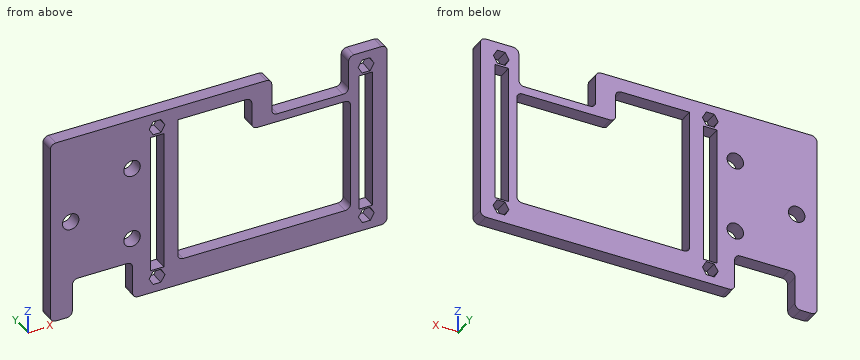
Autodesk Inventor part; units mm, degrees
ref_plane "YZ Plane" through (0, 0, 0) normal (1, 0, 0) x (0, 1, 0)
ref_plane "XZ Plane" through (0, 0, 0) normal (0, 1, 0) x (-1, 0, 0)
ref_plane "XY Plane" through (0, 0, 0) normal (0, 0, 1) x (1, 0, 0)
sketch "Sketch1" plane through (0, 0, 0) normal (0, 1, 0) x (-1, 0, 0)
  line L0 (-2.27, 0) -> (120.44, 0)
  line L1 (120.44, 0) -> (120.44, -68.57)
  line L2 (120.44, -68.57) -> (-2.27, -68.57)
  line L3 (-2.27, -68.57) -> (-2.27, 0)
  line L4 (120.44, -66.57) -> (120.44, -2)
  line L5 (0, -68.57) -> (118.44, -68.57)
  line L6 (-2.27, -2.27) -> (-2.27, -66.3)
  circle A0 centre (81.55, -63.09) radius 1.5
  circle A1 centre (81.55, -63.09) radius 1.5
  line L7 (70.44, -68.57) -> (15.73, -68.57)
  line L8 (51, 0) -> (75, 0)
  line L9 (26, 0) -> (51, 0)
  line L10 (84, -60) -> (79, -60)
  line L11 (79, -60) -> (79, -8.7337)
  line L12 (79, -8.7337) -> (84, -8.7337)
  line L13 (84, -8.7337) -> (84, -60)
  line L14 (8, -60) -> (3, -60)
  line L15 (3, -60) -> (3, -8.7337)
  line L16 (3, -8.7337) -> (8, -8.7337)
  line L17 (8, -8.7337) -> (8, -60)
  circle A2 centre (5.25, -63.09) radius 1.5
  circle A3 centre (5.35, -5.47) radius 1.5
  circle A4 centre (81.55, -5.47) radius 1.5
  circle A5 centre (81.55, -5.47) radius 1.5
  circle A6 centre (5.35, -5.47) radius 1.5
  circle A7 centre (5.25, -63.09) radius 1.5
  dimension "d20" = 3
  dimension "d27" = 3
  dimension "d28" = 3
  dimension "d29" = 3
  dimension "d30" = 68.57
extrude "Extrusion1" add sketch "Sketch1" along normal blind 5
fillet "Fillet4" radius 2 4 edges at (-120.44, 2.5, -68.57) (-120.44, 2.5, 0) (2.27, 2.5, -68.57) (2.27, 2.5, 0)
sketch "Sketch7" plane through (0, 5, 0) normal (0, 1, 0) x (1, 0, 0)
  line L0 (-117.44, 63.57) -> (-87.44, 63.57)
  line L1 (-87.44, 63.57) -> (-87.44, 5)
  line L2 (-87.44, 5) -> (-117.44, 5)
  line L3 (-117.44, 5) -> (-117.44, 63.57)
  line L4 (-120.44, 66.57) -> (-120.44, 2)
  line L5 (0.27, 68.57) -> (-118.44, 68.57)
  line L6 (-118.44, 0) -> (0.27, 0)
  point P0 (0, 0)
  dimension "d67" = 30
  dimension "d68" = 3
  dimension "d69" = 5
  dimension "d70" = 5
extrude "Extrusion6" [suppressed]
fillet "Fillet8" [suppressed]
sketch "Sketch8" plane through (0, 5, 0) normal (0, 1, 0) x (1, 0, 0)
  line L0 (-118.44, 0) -> (0.27, 0)
  line L1 (-39.73, 0) -> (-11.73, 0)
  line L2 (-11.73, 0) -> (-11.73, 14)
  line L3 (-11.73, 14) -> (-39.73, 14)
  line L4 (-39.73, 14) -> (-39.73, 0)
  line L5 (2.27, 2) -> (2.27, 66.57)
  point P0 (0, 0)
  point P1 (-11.73, 0)
  dimension "d74" = 28
  dimension "d75" = 14
  dimension "d82" = 14
extrude "Extrusion7" cut sketch "Sketch8" against normal blind 10
sketch "Sketch9" plane through (0, 5, 0) normal (0, 1, 0) x (1, 0, 0)
  line L0 (-74, 59) -> (-11, 59)
  line L1 (-11, 59) -> (-11, 17)
  line L2 (-11, 17) -> (-74, 17)
  line L3 (-74, 17) -> (-74, 59)
  line L4 (-74, 17) -> (-47.019, 17)
  line L5 (-47.019, 17) -> (-47.019, 5)
  line L6 (-47.019, 5) -> (-74, 5)
  line L7 (-74, 5) -> (-74, 17)
  point P0 (0, 0)
extrude "Extrusion8" cut sketch "Sketch9" against normal blind 5
fillet "Fillet9" radius 2 5 edges at (-74, 2.5, -59) (-11, 2.5, -59) (-11, 2.5, -17) (-47.019, 2.5, -5) (-47.019, 2.5, -17)
fillet "Fillet10" radius 2 4 edges at (-39.73, 2.5, -14) (-11.73, 2.5, -14) (-11.73, 2.5, 0) (-39.73, 2.5, 0)
sketch "Sketch10" plane through (0, 0, 0) normal (0, -1, 0) x (1, 0, 0)
  circle A0 centre (-90.66, -18.55) radius 3
  circle A1 centre (-113.03, -32.07) radius 3
  circle A2 centre (-90.66, -45.53) radius 3
  line L0 (-120.44, -66.57) -> (-120.44, -2)
  line L1 (-118.44, 0) -> (-41.73, 0)
  line L2 (-90.66, -45.53) -> (-90.66, -18.55) construction
  point P0 (0, 0)
  dimension "d83" = 29.78
  dimension "d84" = 18.55
  dimension "d85" = 6
  dimension "d86" = 13.52
  dimension "d87" = 6
  dimension "d88" = 22.37
  dimension "d89" = 13.46
  dimension "d90" = 6
extrude "Extrusion9" cut sketch "Sketch10" against normal blind 10
sketch "Sketch11" plane through (0, 0, 0) normal (0, -1, 0) x (1, 0, 0)
  circle A0 centre (-90.66, -18.55) radius 3
  line L0 (-92.9694, -18.55) -> (-91.8147, -16.55)
  line L1 (-91.8147, -16.55) -> (-89.5053, -16.55)
  line L2 (-89.5053, -16.55) -> (-88.3506, -18.55)
  line L3 (-88.3506, -18.55) -> (-89.5053, -20.55)
  line L4 (-89.5053, -20.55) -> (-91.8147, -20.55)
  line L5 (-91.8147, -20.55) -> (-92.9694, -18.55)
  circle A1 centre (-113.03, -32.07) radius 3
  line L6 (-115.3394, -32.07) -> (-114.1847, -30.07)
  line L7 (-114.1847, -30.07) -> (-111.8753, -30.07)
  line L8 (-111.8753, -30.07) -> (-110.7206, -32.07)
  line L9 (-110.7206, -32.07) -> (-111.8753, -34.07)
  line L10 (-111.8753, -34.07) -> (-114.1847, -34.07)
  line L11 (-114.1847, -34.07) -> (-115.3394, -32.07)
  circle A2 centre (-90.66, -45.53) radius 3
  line L12 (-92.9694, -45.53) -> (-91.8147, -43.53)
  line L13 (-91.8147, -43.53) -> (-89.5053, -43.53)
  line L14 (-89.5053, -43.53) -> (-88.3506, -45.53)
  line L15 (-88.3506, -45.53) -> (-89.5053, -47.53)
  line L16 (-89.5053, -47.53) -> (-91.8147, -47.53)
  line L17 (-91.8147, -47.53) -> (-92.9694, -45.53)
  point P0 (0, 0)
  dimension "d93" = 4
  dimension "d94" = 4
  dimension "d95" = 4
extrude "Extrusion10" [suppressed]
sketch "Sketch12" plane through (0, 0, 0) normal (0, -1, 0) x (1, 0, 0)
  circle A0 centre (-5.35, -5.47) radius 1.5
  line L0 (-8.2368, -5.47) -> (-6.7934, -2.97)
  line L1 (-6.7934, -2.97) -> (-3.9066, -2.97)
  line L2 (-3.9066, -2.97) -> (-2.4632, -5.47)
  line L3 (-2.4632, -5.47) -> (-3.9066, -7.97)
  line L4 (-3.9066, -7.97) -> (-6.7934, -7.97)
  line L5 (-6.7934, -7.97) -> (-8.2368, -5.47)
  circle A1 centre (-81.55, -5.47) radius 1.5
  line L6 (-84.4368, -5.47) -> (-82.9934, -2.97)
  line L7 (-82.9934, -2.97) -> (-80.1066, -2.97)
  line L8 (-80.1066, -2.97) -> (-78.6632, -5.47)
  line L9 (-78.6632, -5.47) -> (-80.1066, -7.97)
  line L10 (-80.1066, -7.97) -> (-82.9934, -7.97)
  line L11 (-82.9934, -7.97) -> (-84.4368, -5.47)
  circle A2 centre (-81.55, -63.09) radius 1.5
  line L12 (-84.4368, -63.09) -> (-82.9934, -60.59)
  line L13 (-82.9934, -60.59) -> (-80.1066, -60.59)
  line L14 (-80.1066, -60.59) -> (-78.6632, -63.09)
  line L15 (-78.6632, -63.09) -> (-80.1066, -65.59)
  line L16 (-80.1066, -65.59) -> (-82.9934, -65.59)
  line L17 (-82.9934, -65.59) -> (-84.4368, -63.09)
  circle A3 centre (-5.25, -63.09) radius 1.5
  line L18 (-6.6934, -60.59) -> (-3.8066, -60.59)
  line L19 (-3.8066, -60.59) -> (-2.3632, -63.09)
  line L20 (-2.3632, -63.09) -> (-3.8066, -65.59)
  line L21 (-3.8066, -65.59) -> (-6.6934, -65.59)
  line L22 (-6.6934, -65.59) -> (-8.1368, -63.09)
  line L23 (-8.1368, -63.09) -> (-6.6934, -60.59)
  line L24 (-8, -60) -> (-3, -60)
  line L25 (-84, -60) -> (-79, -60)
  line L26 (-79, -8.7337) -> (-84, -8.7337)
  line L27 (-3, -8.7337) -> (-8, -8.7337)
  point P0 (0, 0)
  dimension "d98" = 5
  dimension "d99" = 5
  dimension "d100" = 5
extrude "Extrusion11" cut sketch "Sketch12" against normal blind 10
sketch "Sketch13" plane through (0, 5, 0) normal (0, 1, 0) x (1, 0, 0)
  line L0 (0.27, 68.57) -> (-118.44, 68.57)
  line L1 (-112.44, 68.57) -> (-90.44, 68.57)
  line L2 (-90.44, 68.57) -> (-90.44, 54.57)
  line L3 (-90.44, 54.57) -> (-112.44, 54.57)
  line L4 (-112.44, 54.57) -> (-112.44, 68.57)
  line L5 (-120.44, 66.57) -> (-120.44, 2)
  point P0 (0, 0)
  point P1 (-90.44, 68.57)
  dimension "d103" = 8
  dimension "d104" = 22
  dimension "d105" = 14
extrude "Extrusion12" cut sketch "Sketch13" against normal blind 10
fillet "Fillet11" radius 2 4 edges at (-112.44, 2.5, -68.57) (-90.44, 2.5, -68.57) (-112.44, 2.5, -54.57) (-90.44, 2.5, -54.57)
properties part number "Middle PMMA"
Input: part model. Units: mm. Frame: model coordinates. Give positions to 0.01 mm unless a question says otherwise; leave off trailing zeros. Order: outer loops, then holes, each group sorted by start corner. A loop starts at its lowest first (then second) coordinate and runs counter-clockwise, first axis right, second up. Notation, with made-up numbers: (88.25, 55) - (145.25, 55) arc R24 ccw to (145.25, 88) - close; hole circle Ø8 at (75, -35.5). An arc over 180 degrees is marked (long way). Put each result on its own line as item: value.
Item 1: Contact query for flat-ended pins moving along their axis: pin 1 (1.5 mm diameter, centred on x = -34.5, y = 2.5, fed in from +Z); pin 2 (9.5 mm diameter, centred on x = -113.03, z = -32.07, fed in from -Y). Output: stop coordinate, or through.
Found:
pin 1: stops at z = -14
pin 2: stops at y = 0
Item 2: Ray query, L1, parallel to X at y = 1.6, z = -11; L2, parallel to X at y = 0.7, z = -26; L3, parallel to Z at x = -51, y = 0.65. Return the intervals inside material, ascending. Write a range as from..to.
Found:
L1: x = -120.44..-84, -79..-74, -47.02..-39.73, -11.73..-8, -3..2.27
L2: x = -120.44..-84, -79..-74, -11..-8, -3..2.27
L3: z = -68.57..-59, -5..0
Item 3: Section query A-A, the plane z = -38. Return loops of the section in (x, y).
Found:
outline: (-120.44, 0) - (-84, 0) - (-84, 5) - (-120.44, 5) - close; (-79, 0) - (-74, 0) - (-74, 5) - (-79, 5) - close; (-11, 0) - (-8, 0) - (-8, 5) - (-11, 5) - close; (-3, 0) - (2.27, 0) - (2.27, 5) - (-3, 5) - close
Item 4: Section query B-B, the plane z = -45.53. Return loops of the section in (x, y).
Found:
outline: (-120.44, 0) - (-93.66, 0) - (-93.66, 5) - (-120.44, 5) - close; (-87.66, 0) - (-84, 0) - (-84, 5) - (-87.66, 5) - close; (-79, 0) - (-74, 0) - (-74, 5) - (-79, 5) - close; (-11, 0) - (-8, 0) - (-8, 5) - (-11, 5) - close; (-3, 0) - (2.27, 0) - (2.27, 5) - (-3, 5) - close
Item 5: Section query C-C, the plane y = 3.75. Count the separate pieces of the cut face and the enclosed holes in it, then the cut area to 3 significant figures.
Found:
separate pieces: 1
enclosed holes: 10
area: 4,060 mm^2
